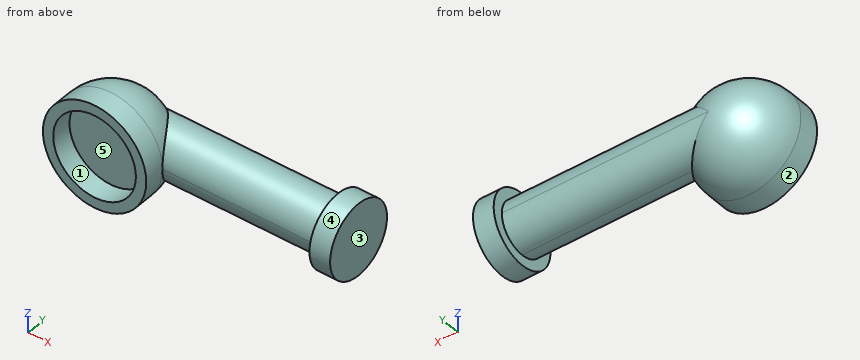
```python
from build123d import *

# Parameters (mm, degrees)
SKETCH_1_R      = 2.5
SKETCH_1_R_2    = 2
EXTRUDE_1_DEPTH = 1
EXTRUDE_2_DEPTH = 10
SKETCH_4_R      = 1.75
EXTRUDE_3_DEPTH = 1


with BuildPart() as part:
    # Sketch 1 → Extrude 1 (new body)
    with BuildSketch(Plane(origin=(0, 0, 0), x_dir=(1, 0, 0), z_dir=(0, 1, 0))):
        Circle(SKETCH_1_R)
        Circle(SKETCH_1_R_2, mode=Mode.SUBTRACT)
    extrude(amount=EXTRUDE_1_DEPTH)

    # Sketch 2 → Revolve 1 (revolve)
    with BuildSketch(Plane.XY):
        with BuildLine():
            Line((0, 1), (2.5, 1))
            ThreePointArc((2.5, 1), (1.767766953, 2.767766953), (0, 3.5))
            Line((0, 3.5), (0, 1))
        make_face()
    revolve(axis=Axis((0, 1, 0), (0, 1, 0)))

    # Sketch 3 → Extrude 2 (add)
    with BuildSketch(Plane(origin=(0, 0, 0), x_dir=(0, 0, -1), z_dir=(1, 0, 0))):
        with BuildLine():
            ThreePointArc((0, 3.5), (-1.25, 2.25), (0, 1))
            Line((0, 1), (0, 3.5))
        make_face()
        with BuildLine():
            Line((0, 3.5), (0, 1))
            ThreePointArc((0, 1), (0.883883476, 1.366116524), (1.25, 2.25))
            ThreePointArc((1.25, 2.25), (0.883883476, 3.133883476), (0, 3.5))
        make_face()
    extrude(amount=EXTRUDE_2_DEPTH)

    # Sketch 4 → Extrude 3 (add)
    with BuildSketch(Plane(origin=(10, 0, 0), x_dir=(0, 0, -1), z_dir=(1, 0, 0))):
        with Locations((0, 2.25)):
            Circle(SKETCH_4_R)
    extrude(amount=EXTRUDE_3_DEPTH)


solid = part.part
```
Design review of the part built by this model. Coordinates are the model's own, in mm. Face numbers are marked on the shaded views. A direction names the side the tool comes from. Give positions to 0.01 mm unless a question says otherwise; leave off trailing zeros. Loops run counter-clockwise (first coordinate to the right, second up) from the corner with the lowest first, then second, coordinate; pieces in that order, holes last. Notation, with made-up numbers: M 42.25,64 L 66.25,64 A28 cw 66.25,102 Z; hole C -26.75,-19.5 d6. An arc over 180 degrees is marked long. Return JSON: item names as keys, results as strings. Group by question number.
Item 1: Mouldability with a two-part tool opening along Z and no side actions: class the marked faces 1, 2 and 3 as released by +Z, released by -Z, zero draft, split by the parting line, or undercut.
Item 2: We need section A-A (y = 1.2). Give the boundary of the cut face in (x, z), and give its area (3 significant figures).
Item 3: Tool access review of the marked faces 4 and 5: name each direction out of +Z, -Z, +X, -X, +Y, -Y from which nothing blocks a thin tool from reaching the whole face with its end or side.
Item 4: We need section B-B (x = -0.5). Give the boundary of the cut face in (y, z).
Item 5: Insertion check: pin 1 Ø3 at (x, z) = (0, 1.5) entering from -Y; pin 2 Ø3 at (x, z) = (1.5, 0) entering from +Y; pin 3 Ø1 at (x, z) = (5, -2) entering from -Y; pin 4 Ø2 at (y, z) = (2.5, 0) entering from -X. Each pin has a flat end and moves straight along its axis. Give the tip position at first contact, or say it passes through.
Item 6: We need section C-C (x = 6.5). Give the boundary of the cut face in (y, z), and give its area (3 significant figures).
Item 7: For probe 1 along X at (y, z) = (0.7, 0); probe 2 along Z at (x, y) = (0, 0.6), list the stretches that pass through material, from the lowest coordinate up.
Output:
{
 "1": {"face 1": "undercut", "face 2": "split by the parting line", "face 3": "zero draft"},
 "2": {"outline": "M 2.4,-0.68 L 10,-0.68 L 10,-1.4 L 11,-1.4 L 11,1.4 L 10,1.4 L 10,0.68 L 2.4,0.68 A2.49 ccw long Z", "area": "32.5 mm^2"},
 "3": {"face 4": "+X", "face 5": "-Y"},
 "4": {"outline": "M 0,-2.45 L 1,-2.45 A2.45 ccw 1,2.45 L 0,2.45 L 0,1.94 L 1,1.94 L 1,-1.94 L 0,-1.94 Z"},
 "5": {"pin 1": "stops at y = 0", "pin 2": "stops at y = 3.5", "pin 3": "passes through", "pin 4": "stops at x = -2.45"},
 "6": {"outline": "C 2.25,0 d2.5", "area": "4.91 mm^2"},
 "7": {"probe 1": "x = -2.5 to -2, 2 to 2.5, 10 to 11", "probe 2": "z = -2.5 to -2, 2 to 2.5"}
}
